For this review, take the finished solid that the model builds, in its own axes (mm). A direction names the side the tool comes from. Coordinates: 2 decimals unless noted, no trailing zeros. Write each loop counter-clockwise with the first axis right and the second up, starting at its lowest first coordinate (ties: lowest second). Pieces come first, ordered by that corner, then holes. Notation, with made-up numbers: M -15,79 L 5,79 A9 ccw 5,86 Z; hole C 57,68 d11. An arc over 180 degrees is marked long. One line per question, with ' | ' between items.
Autodesk Inventor part; units mm, degrees
ref_plane "YZ Plane" through (0, 0, 0) normal (1, 0, 0) x (0, 1, 0)
ref_plane "XZ Plane" through (0, 0, 0) normal (0, 1, 0) x (-1, 0, 0)
ref_plane "XY Plane" through (0, 0, 0) normal (0, 0, 1) x (1, 0, 0)
sketch "Sketch1" plane through (0, 0, 0) normal (0, 1, 0) x (-1, 0, 0)
  line L0 (13.8, 22.25) -> (-13.8, 22.25)
  line L1 (-23.8, 12.25) -> (-23.8, -12.25)
  line L2 (-13.8, -22.25) -> (13.8, -22.25)
  line L3 (23.8, -12.25) -> (23.8, 12.25)
  line L4 (23.8, 22.25) -> (-23.8, -22.25) construction
  line L5 (-23.8, 22.25) -> (23.8, -22.25) construction
  arc A0 (23.8, 12.25) -> (13.8, 22.25) centre (13.8, 12.25) ccw
  arc A1 (13.8, -22.25) -> (23.8, -12.25) centre (13.8, -12.25) ccw
  arc A2 (-23.8, -12.25) -> (-13.8, -22.25) centre (-13.8, -12.25) ccw
  arc A3 (-13.8, 22.25) -> (-23.8, 12.25) centre (-13.8, 12.25) ccw
  point P0 (0, 0)
  dimension "d0" = 47.6
  dimension "d1" = 44.5
  dimension "d3" = 10
extrude "Extrusion1" add sketch "Sketch1" along normal blind 8.25
fillet "Fillet1" radius 1 16 edges at (20.8711, 0, 19.3211) (23.8, 0, 0) (20.8711, 0, -19.3211) (0, 0, -22.25) (-20.8711, 0, -19.3211) (-23.8, 0, 0) (-20.8711, 0, 19.3211) (0, 0, 22.25) (23.8, 8.25, 0) (20.8711, 8.25, -19.3211) (0, 8.25, -22.25) (-20.8711, 8.25, -19.3211) (-23.8, 8.25, 0) (-20.8711, 8.25, 19.3211) (0, 8.25, 22.25) (20.8711, 8.25, 19.3211)
sketch "Sketch2" plane through (0, 0, 0) normal (0, -1, 0) x (1, 0, 0)
  line L0 (-33.32, 0) -> (33.32, 0)
  line L1 (0, -31.15) -> (0, 31.15)
  point P0 (0, 0)
  point P1 (17, 12.5)
  point P2 (17, -12.5)
  point P3 (-17, 12.5)
  point P4 (-17, -12.5)
  dimension "d7" = 25
  dimension "d8" = 34
sketch "Sketch3" plane through (0, 0, 0) normal (0, -1, 0) x (1, 0, 0)
  line L0 (1.3258, -1.3258) -> (-1.3258, 1.3258) construction
  line L1 (1.7678, -0.8839) -> (-0.8839, 1.7678)
  line L2 (-1.7678, 0.8839) -> (0.8839, -1.7678)
  arc A0 (0.8839, -1.7678) -> (1.7678, -0.8839) centre (1.3258, -1.3258) ccw
  arc A1 (-0.8839, 1.7678) -> (-1.7678, 0.8839) centre (-1.3258, 1.3258) ccw
  line L3 (0, -31.15) -> (0, 31.15)
  point P0 (0, 0)
  point P1 (-1.7678, 1.7678)
  point P2 (1.7678, -1.7678)
  dimension "d9" = 5
  dimension "d10" = 1.25
  dimension "d11" = 135
extrude "Extrusion2" cut sketch "Sketch3" against normal blind 0.5
sketch "Sketch5" plane through (0, 8.25, 0) normal (0, 1, 0) x (1, 0, 0)
  line L0 (15, 10) -> (15, -10) construction
  line L1 (11.5, 10) -> (11.5, -10)
  line L2 (18.5, -10) -> (18.5, 10)
  arc A0 (18.5, 10) -> (11.5, 10) centre (15, 10) ccw
  arc A1 (11.5, -10) -> (18.5, -10) centre (15, -10) ccw
  point P0 (0, 0)
  point P1 (15, 0)
  dimension "d16" = 10
  dimension "d17" = 7
  dimension "d18" = 15
extrude "Extrusion4" add sketch "Sketch5" along normal blind 1
properties part number "Pin-Low-Fidelity"
1) We need section C-C on z = -4. State the section outline as (x, y) points, then the cut area to 3 significant figures.
Responses:
outline: M -23.8,1 A1 ccw -22.8,0 L 22.8,0 A1 ccw 23.8,1 L 23.8,7.25 A1 ccw 22.8,8.25 L 18.5,8.25 L 18.5,9.25 L 11.5,9.25 L 11.5,8.25 L -22.8,8.25 A1 ccw -23.8,7.25 Z | area: 399 mm^2
2) We need section A-A on y = 5.5. State the section outline as (x, z) points.
Responses:
outline: M -23.8,-12.25 A10 ccw -13.8,-22.25 L 13.8,-22.25 A10 ccw 23.8,-12.25 L 23.8,12.25 A10 ccw 13.8,22.25 L -13.8,22.25 A10 ccw -23.8,12.25 Z
3) Machinability: for faces 5 (the flat face through (18.5, 9, 0)), 6 (the flat face through (-0.461, 0.246, -0.423)), 7 (the cylindrical face through (14.9, 8.7, -13.5)), 8 (the cylindrical face through (15.1, 8.7, 13.5)), 9 (the flat face through (11.5, 9, 0)), which of the approach directions +Z, -Z, +X, -X, +Y, -Y give a long, thin tool a straight path to every point of the face, cutting with its end or side? Answer none if there is none.
Responses:
face 5: +Z, -Z, +X, +Y | face 6: -Y | face 7: -Z, +Y | face 8: +Z, +Y | face 9: +Z, -Z, -X, +Y
4) We need section B-B on x = -2.5. State the section outline as (y, z) points, then the cut area to 3 significant figures.
Responses:
outline: M 0,-21.25 A1 ccw 1,-22.25 L 7.25,-22.25 A1 ccw 8.25,-21.25 L 8.25,21.25 A1 ccw 7.25,22.25 L 1,22.25 A1 ccw 0,21.25 Z | area: 366 mm^2
5) The part is to be moulded in two halves that separate along X. For faces 1 (the cylindrical face through (20.95, 4.08, 19.24)), 2 (the cylindrical face through (-1.758, 0.246, 1.777)), 3 (the cylindrical face through (-23.515, 0.301, 0.172)), 4 (the cylindrical face through (0.193, 7.965, 21.949)), say which applies: +X half, -X half, draft (parallel to the pull), parting line (faces both ways), or undercut.
Responses:
face 1: +X half | face 2: undercut | face 3: -X half | face 4: draft
6) Insertion check: pin 1 Ø1.5 at (x, y) = (-17, 4.5) entering from +Z. The pin has a flat end and moves straight along its axis. Give the tip position at first contact, or say it passes through.
Responses:
pin 1: z = 21.95
7) To check wall thickness, follow line 1 along Y through (x, z) = (1, 1); line 2 along X through (y, z) = (3.5, 18); line 3 along Z through (x, y) = (18.5, 7.5). State the ranges of each line that lie inside material, in increasing order. Write a range as [from, to].
Responses:
line 1: [0, 8.25] | line 2: [-21.98, 21.98] | line 3: [-21.04, 21.04]
